Could you check a few things on this drawing? It's one solid part, dimensions in mm from its lowest x, y, z. Give positions to 0.01 mm unless a question says otherwise; leave off trailing zeros. Order: outer loops, then holes, each group sorted by start corner. A loop starts at its lowest first (then second) coordinate and runs counter-clockwise, first axis right, second up. Notation, with made-up numbers: (67, 74) -> (72, 74) arc R19 cw to (72, 100) -> close; hole circle Ø5 at (-4, 67.25). An arc over 180 degrees is marked (long way). Answer as a JSON object with one key per item and string values.
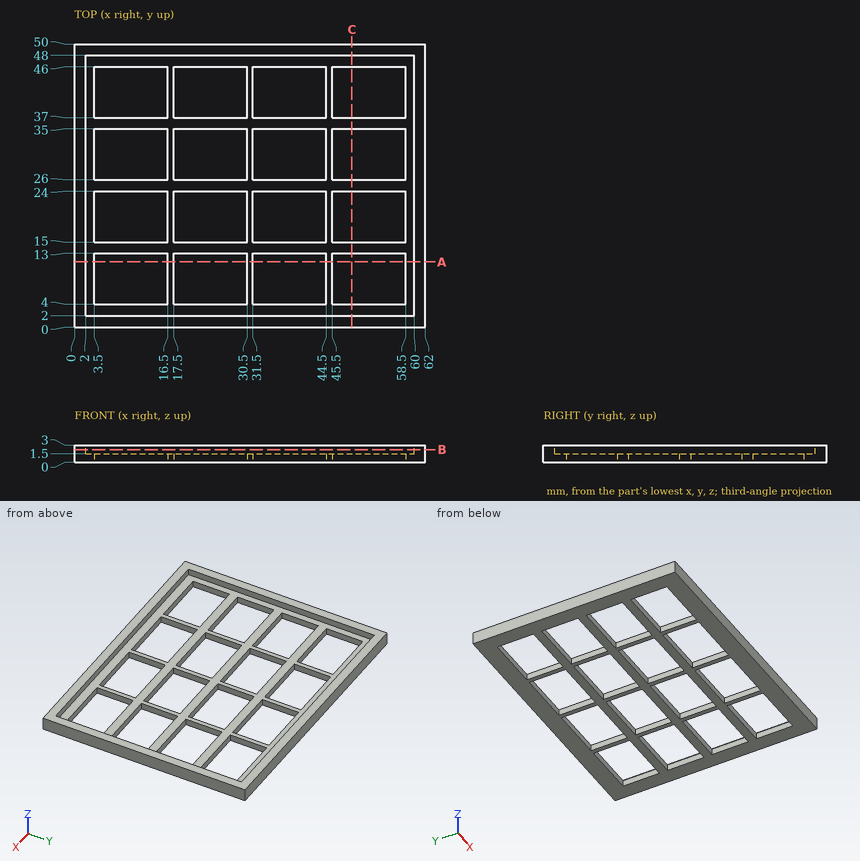
1. If we section it at A-A on y = 11.5: Please give me the cut outline in (x, z), then the cut area to 3 significant figures.
Worked answers:
{"outline": "(0, 0) -> (3.5, 0) -> (3.5, 1.5) -> (2, 1.5) -> (2, 3) -> (0, 3) -> close; (16.5, 0) -> (17.5, 0) -> (17.5, 1.5) -> (16.5, 1.5) -> close; (30.5, 0) -> (31.5, 0) -> (31.5, 1.5) -> (30.5, 1.5) -> close; (44.5, 0) -> (45.5, 0) -> (45.5, 1.5) -> (44.5, 1.5) -> close; (58.5, 0) -> (62, 0) -> (62, 3) -> (60, 3) -> (60, 1.5) -> (58.5, 1.5) -> close", "area": "21.0 mm²"}
2. Will this pin go through, and if not, where does the flat tip stop? pin 1 Ø1.5 at (x, y) = (11.5, 39.5) entering from -Z.
Worked answers:
{"pin 1": "through"}
3. If we section it at C-C on x = 49: Please give me the cut outline in (y, z), then the cut area to 3 significant figures.
Worked answers:
{"outline": "(0, 0) -> (4, 0) -> (4, 1.5) -> (2, 1.5) -> (2, 3) -> (0, 3) -> close; (13, 0) -> (15, 0) -> (15, 1.5) -> (13, 1.5) -> close; (24, 0) -> (26, 0) -> (26, 1.5) -> (24, 1.5) -> close; (35, 0) -> (37, 0) -> (37, 1.5) -> (35, 1.5) -> close; (46, 0) -> (50, 0) -> (50, 3) -> (48, 3) -> (48, 1.5) -> (46, 1.5) -> close", "area": "27.0 mm²"}
4. If we section it at B-B on z = 2.2: Please give me the cut outline in (x, y).
Worked answers:
{"outline": "(0, 0) -> (62, 0) -> (62, 50) -> (0, 50) -> close; hole (2, 2) -> (60, 2) -> (60, 48) -> (2, 48) -> close"}
5. Please list where these lines run through material, in increasing order: L1, parallel to Y at x = 8.5, z = 1.4; L2, parallel to X at y = 23, z = 0.25; L3, parallel to X at y = 12, z = 1.75.
Worked answers:
{"L1": "0 to 4, 13 to 15, 24 to 26, 35 to 37, 46 to 50", "L2": "0 to 3.5, 16.5 to 17.5, 30.5 to 31.5, 44.5 to 45.5, 58.5 to 62", "L3": "0 to 2, 60 to 62"}
